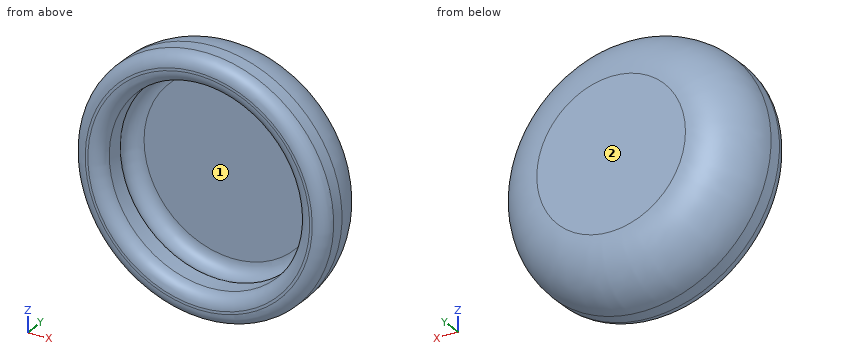
from build123d import *


with BuildPart() as part:
    # Sketch3 → Revolve1 (revolve)
    with BuildSketch(Plane(origin=(0, 0, 0), x_dir=(0, 0, -1), z_dir=(1, 0, 0))):
        with BuildLine():
            Line((12.319000296, -5.080996249), (12.319000296, -6.349750932))
            ThreePointArc((12.319000296, -6.349750932), (11.946952958, -7.247952662), (11.048751227, -7.62))
            Line((11.048751227, -7.62), (10.795249364, -7.62))
            ThreePointArc((10.795249364, -7.62), (9.897047634, -7.247952662), (9.525000296, -6.349750932))
            Line((9.525000296, -6.349750932), (9.525000296, -4.68336138))
            ThreePointArc((9.525000296, -4.68336138), (9.684048002, -3.333611598), (8.534504688, -2.60858))
            Line((8.534504688, -2.60858), (0, -2.60858))
            Line((0, -2.60858), (0, 0))
            Line((0, 0), (7.238004047, 0))
            ThreePointArc((7.238004047, 0), (10.83081095, -1.488189346), (12.319000296, -5.080996249))
        make_face()
    revolve(axis=Axis((0, -2.60858, 0), (0, -1, 0)))


solid = part.part
Can you work these out from the model? Positions are in its coordinate system, mm. Face numbers are marked on the shaded views. Coordinates: 2 decimals unless noted, no trailing zeros. Write each loop counter-clockwise with the first axis right and the second up, starting at its lowest first coordinate (ties: lowest second). Pieces come first, ordered by that corner, then holes. Notation, with made-up numbers: (24.25, -33.75) - (83.25, -33.75) arc R21 cw to (83.25, -25.75) - close; hole circle Ø6 at (71.5, 71.5). An arc over 180 degrees is marked (long way). Return JSON: item names as keys, results as strings. Group by question number.
Item 1: I'm going to push flat-ended pins straight in: pin 1 Ø11.5 at (x, z) = (0, 0) entering from -Y; pin 2 Ø1.5 at (x, z) = (-9.5, -5) entering from +Y; pin 3 Ø4 at (y, z) = (-4, -4) entering from -X. Where does each tip first touch, or does it pass through?
Item 2: Please list where these lines run through material, in increasing order: probe 1 along X at (y, z) = (-5.8, 0) (3 decimals); probe 2 along X at (y, z) = (-6.75, -4.75); probe 3 along Y at (x, z) = (-4.75, 1.5).
Item 3: We'd pull the mould along Z, two halves only. Please class the marked faces 1 and 2: pulls with the +Z half, pulls with the -Z half, needs draft (parallel to the pull), parting line crosses it, or undercut.
Item 4: If we section it at D-D (y = -1.5): Write out the boundary of the cut face in (x, z).
Item 5: If we section it at C-C (y = -5.5): Write out the boundary of the cut face in (x, z) (3 decimals), then the cut area to 3 significant figures.
Return value:
{
 "1": {"pin 1": "stops at y = -2.61", "pin 2": "stops at y = -0.81", "pin 3": "stops at x = -12.12"},
 "2": {"probe 1": "x = -12.319 to -9.525, 9.525 to 12.319", "probe 2": "x = -11.3 to -8.33, 8.33 to 11.3", "probe 3": "y = -2.61 to 0"},
 "3": {"face 1": "undercut", "face 2": "needs draft"},
 "4": {"outline": "circle Ø21.69 at (0, 0)"},
 "5": {"outline": "circle Ø24.638 at (0, 0); hole circle Ø19.05 at (0, 0)", "area": "192 mm^2"}
}
